Autodesk Inventor part; units mm, degrees
ref_plane "YZ Plane" through (0, 0, 0) normal (1, 0, 0) x (0, 1, 0)
ref_plane "XZ Plane" through (0, 0, 0) normal (0, 1, 0) x (-1, 0, 0)
ref_plane "XY Plane" through (0, 0, 0) normal (0, 0, 1) x (1, 0, 0)
sketch "Sketch1" plane through (0, 0, 0) normal (0, 1, 0) x (-1, 0, 0)
  line L0 (41.1155, 0) -> (-17.3761, 27.2751)
  line L1 (-17.3761, 27.2751) -> (-17.3761, -27.2751)
  line L2 (-17.3761, -27.2751) -> (41.1155, 0)
  circle A0 centre (-6.4761, -10.1655) radius 10.9
  circle A1 centre (-6.4761, 10.1655) radius 10.9
  circle A2 centre (15.3239, 0) radius 10.9
  circle A3 centre (0, 0) radius 17.3761
  line L3 (52.8138, 0) -> (-29.0745, 0)
  point P0 (-1.8696, 20.0443)
  point P1 (-17.3761, 10.1655)
  point P2 (-17.3761, -10.1655)
  point P3 (-1.8696, -20.0443)
  point P4 (19.9304, -9.8788)
  point P5 (19.9304, 9.8788)
  dimension "d0" = 50
  dimension "d1" = 21.8
  dimension "d2" = 32.7
  dimension "d3" = 21.8
  dimension "d4" = 21.8
extrude "Extrusion1" add sketch "Sketch1" along normal blind 1 contours A2 A3 L0 | A2 L3 A3 | L2 A3 A2 | A2 A3 L3 | A3 A1 L0 | A3 A2 L3 A1 | A3 L3 A2 | L2 A0 A3 | A3 A0 L3 A2 | A2 L3 A3 | A1 A3 | A1 A0 A3 | A0 A3 | A3 A0 A1 | A1 A3 L1 | A1 L3 A3 | L3 A0 | A1 L3 | L1 A3 A0 | A3 L3 A0
sketch "Sketch2" plane through (0, 1, 0) normal (0, 1, 0) x (1, 0, 0)
  line L0 (17.3761, -10.1655) -> (17.3761, 10.1655)
  arc A0 (17.3761, 10.1655) -> (1.8696, 20.0443) centre (6.4761, 10.1655) ccw
  line L1 (1.8696, 20.0443) -> (-19.9304, 9.8788)
  arc A1 (-19.9304, 9.8788) -> (-19.9304, -9.8788) centre (-15.3239, 0) ccw
  line L2 (-19.9304, -9.8788) -> (1.8696, -20.0443)
  arc A2 (1.8696, -20.0443) -> (17.3761, -10.1655) centre (6.4761, -10.1655) ccw
  circle A3 centre (-15.3239, 0) radius 11.336
  circle A4 centre (6.4761, -10.1655) radius 11.336
  circle A5 centre (6.4761, 10.1655) radius 11.336
  line L3 (-20.1147, -10.2739) -> (1.6853, -20.4394)
  line L4 (-20.1147, 10.2739) -> (1.6853, 20.4394)
  line L5 (17.8121, -26) -> (17.8121, 10.1655)
  point P0 (0, 0)
  point P1 (17.8121, -10.1655)
  dimension "d9" = 22.672
  dimension "d7" = 22.672
  dimension "d8" = 22.672
extrude "Extrusion2" add sketch "Sketch2" against normal blind 1
sketch "Sketch3" plane through (0, 0, 0) normal (0, -1, 0) x (1, 0, 0)
  arc A0 (1.6853, -20.4394) -> (17.8121, -10.1655) centre (6.4761, -10.1655) ccw
  line L0 (17.8121, -10.1655) -> (17.8121, 10.1655)
  arc A1 (17.8121, 10.1655) -> (1.6853, 20.4394) centre (6.4761, 10.1655) ccw
  line L1 (1.6853, 20.4394) -> (-20.1147, 10.2739)
  arc A2 (-20.1147, 10.2739) -> (-20.1147, -10.2739) centre (-15.3239, 0) ccw
  line L2 (-20.1147, -10.2739) -> (1.6853, -20.4394)
  circle A3 centre (-15.3239, 0) radius 10.236
  circle A4 centre (6.4761, 10.1655) radius 10.236
  circle A5 centre (6.4761, -10.1655) radius 10.236
  line L3 (-19.6498, -9.277) -> (2.1502, -19.4425)
  line L4 (16.7121, -10.1655) -> (16.7121, 10.1655)
  line L5 (-19.6498, 9.277) -> (2.1502, 19.4425)
  point P0 (0, 0)
  point P1 (-8.7498, -14.3597)
  dimension "d17" = 1.1
extrude "Extrusion3" add sketch "Sketch3" along normal blind 5.1
sketch "Sketch4" plane through (0, -5.1, 0) normal (0, -1, 0) x (1, 0, 0)
  line L0 (1.6853, 20.4394) -> (-20.1147, 10.2739)
  arc A0 (17.8121, 10.1655) -> (1.6853, 20.4394) centre (6.4761, 10.1655) ccw
  line L1 (17.8121, -10.1655) -> (17.8121, 10.1655)
  arc A1 (1.6853, -20.4394) -> (17.8121, -10.1655) centre (6.4761, -10.1655) ccw
  line L2 (-20.1147, -10.2739) -> (1.6853, -20.4394)
  arc A2 (-20.1147, 10.2739) -> (-20.1147, -10.2739) centre (-15.3239, 0) ccw
  circle A3 centre (6.4761, -10.1655) radius 6.136
  circle A4 centre (6.4761, 10.1655) radius 6.136
  circle A5 centre (-15.3239, 0) radius 6.136
  line L3 (-17.917, -5.5611) -> (3.883, -15.7266)
  line L4 (12.6121, -10.1655) -> (12.6121, 10.1655)
  line L5 (3.883, 15.7266) -> (-17.917, 5.5611)
  point P0 (0, 0)
  dimension "d18" = 5.2
extrude "Extrusion4" add sketch "Sketch4" along normal blind 1.1
properties part number "Magne_Cover"
Here's how the part is built. I have some questions about the finished solid (model axes, mm). A direction names the side the tool comes from. Round coordinates to 2 decimals unless told otherwise and drop trailing zeros. Loops run counter-clockwise (first coordinate to the right, second up) from the corner with the lowest first, then second, coordinate; pieces in that order, holes last.
1. Thinking about a two-plate mould opening in X: for faces 4 (the face through (17.812, -3, 0)), 5 (the face through (-8, -6.2, -13)), 6 (the face through (0, 0, 0)), which applies, released by +X, released by -X, zero draft, split by the parting line, or undercut?
Answers:
face 4: released by +X
face 5: zero draft
face 6: undercut
2. For faces 1 (the face through (-9.367, -2.55, -15.285)), 2 (the face through (9.7, -5.642, 15.386)), 3 (the face through (12.1, -2.51, -18.72)), which set-ups out of +Z, -Z, +X, -X, +Y, -Y let a thin tool reach every point of the face, with its end or its side?
Answers:
face 1: -Z, -X, +Y, -Y
face 2: -Y
face 3: none
3. Suppose I cut it at B-B, the plane y = -4.5. Please give me the cut outline in (x, z).
Answers:
outline: (-20.11, -10.27) - (1.69, -20.44) arc R11.34 ccw to (17.81, -10.17) - (17.81, 10.17) arc R11.34 ccw to (1.69, 20.44) - (-20.11, 10.27) arc R11.34 ccw to start; hole (-19.65, -9.28) - (2.15, -19.44) arc R10.24 ccw to (16.71, -10.17) - (16.71, 10.17) arc R10.24 ccw to (2.15, 19.44) - (-19.65, 9.28) arc R10.24 ccw to start
4. If I drill on probe 1 along Z at (x, y) = (6.5, -2.25); probe 2 along Y at (x, z) = (0, -18); probe 3 along Y at (x, z) = (6, 0), over which ranges is the centre line in solid material (lowest first)?
Answers:
probe 1: z = -21.5 to -20.4, 20.4 to 21.5
probe 2: y = -6.2 to -5.1, 0 to 1
probe 3: y = 0 to 1
5. Suppose I cut it at D-D, the plane x = -14. Please give me the cut outline in (y, z), and give its area (3 significant figures).
Answers:
outline: (-6.2, -13.13) - (1, -13.13) - (1, 13.13) - (-6.2, 13.13) - (-6.2, 7.39) - (-5.1, 7.39) - (-5.1, 11.91) - (0, 11.91) - (0, -11.91) - (-5.1, -11.91) - (-5.1, -7.39) - (-6.2, -7.39) - close
area: 51.3 mm2
6. Suppose I cut it at C-C, the plane x = 13.5. Please give me the cut outline in (y, z), and give its area (3 significant figures).
Answers:
outline: (-6.2, -19.06) - (1, -19.06) - (1, 19.06) - (-6.2, 19.06) - close; hole (-5.1, -17.61) - (0, -17.61) - (0, 17.61) - (-5.1, 17.61) - close
area: 94.9 mm2
7. Suppose I cut it at A-A, the plane z = 17.5. Please give me the cut outline in (x, y).
Answers:
outline: (-4.62, -6.2) - (15.12, -6.2) - (15.12, 1) - (-4.62, 1) - close; hole (-2.02, -5.1) - (13.62, -5.1) - (13.62, 0) - (-2.02, 0) - close
8. Will these pins go through, and if not, where does the flat tip stop? pin 1 (1.5 mm diameter, centred on x = -3, y = -3.5, fed in from +Z); pin 2 (1.2 mm diameter, centred on y = -5.5, z = -4, fed in from -X); pin 3 (1.5 mm diameter, centred on x = -4.5, y = -3, fed in from +Z).
Answers:
pin 1: stops at z = 18.6
pin 2: stops at x = -26.14
pin 3: stops at z = 17.9
